CAD build for the part. Positions are in the model's coordinates, mm. Give positions to 0.01 mm unless a question says otherwise; leave off trailing zeros. Write each loop counter-clockwise with the first axis right and the second up, starting at its lowest first coordinate (ties: lowest second). Pieces come first, ordered by that corner, then holes. Notation, with made-up numbers: (43.25, 70) - (63.25, 70) arc R35 ccw to (63.25, 104) - close; hole circle Ø7 at (74.5, -21.75). An arc over 180 degrees is marked (long way). Answer as a JSON object with one key per item and string values.
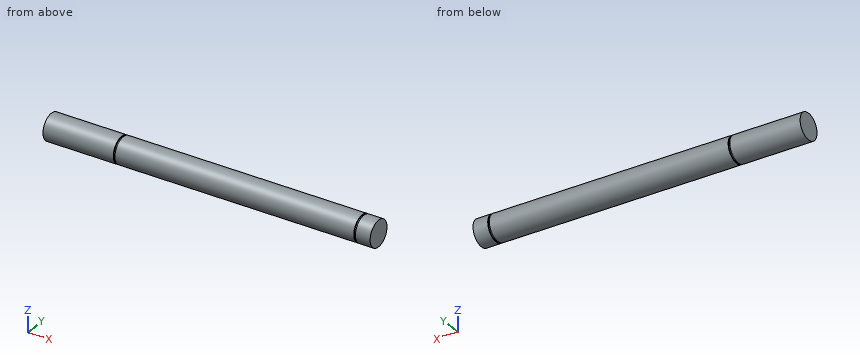
from build123d import *

# Parameters (mm, degrees)
SKETCH1_R           = 4
BOSS_EXTRUDE1_DEPTH = 50
SKETCH2_W           = 0.5
SKETCH2_H           = 0.3
SKETCH3_W           = 0.5
SKETCH3_H           = 0.3


with BuildPart() as part:
    # Sketch1 → Boss-Extrude1 (new, symmetric)
    with BuildSketch(Plane(origin=(0, 0, 0), x_dir=(0, 0, -1), z_dir=(1, 0, 0))):
        Circle(SKETCH1_R)
    extrude(amount=BOSS_EXTRUDE1_DEPTH, both=True)

    # Sketch2 → Cut-Revolve1 (revolve, cut)
    with BuildSketch(Plane.XY, mode=Mode.PRIVATE) as cut_revolve1_sk:
        with Locations((45.25, 3.85)):
            Rectangle(SKETCH2_W, SKETCH2_H)
    revolve(cut_revolve1_sk.sketch.rotate(Axis((0, 0, 0), (1, 0, 0)), 90), axis=Axis((0, 0, 0), (1, 0, 0)), mode=Mode.SUBTRACT)

    # Sketch3 → Cut-Revolve2 (revolve, cut)
    with BuildSketch(Plane.XY, mode=Mode.PRIVATE) as cut_revolve2_sk:
        with Locations((-28.25, 3.85)):
            Rectangle(SKETCH3_W, SKETCH3_H)
    revolve(cut_revolve2_sk.sketch.rotate(Axis((0, 0, 0), (-1, 0, 0)), 270), axis=Axis((0, 0, 0), (-1, 0, 0)), mode=Mode.SUBTRACT)


solid = part.part
(1) Flat gauge pin, fed straight in: P1, Ø1, axis at x = 28.5, z = -2, coming from the -Y side. Where does the tip first touch, or does it go through?
Answer key:
{"P1": "stops at y = -3.71"}
(2) Saw through at A-A, the plane y = -1.5. Give the cut face in (x, z), and give its area (3 significant figures).
Answer key:
{"outline": "(-50, -3.71) - (-28.5, -3.71) - (-28.5, -3.38) - (-28, -3.38) - (-28, -3.71) - (45, -3.71) - (45, -3.38) - (45.5, -3.38) - (45.5, -3.71) - (50, -3.71) - (50, 3.71) - (45.5, 3.71) - (45.5, 3.38) - (45, 3.38) - (45, 3.71) - (-28, 3.71) - (-28, 3.38) - (-28.5, 3.38) - (-28.5, 3.71) - (-50, 3.71) - close", "area": "741 mm²"}
(3) Probe L1, parallel to X at y = -1, z = 3.75; L2, parallel to Z at x = -38.5, y = 0.25; L3, parallel to Z at x = 38, y = -1.5. List the from-to ranges inside material, lowest first. Write a range as [from, to].
Answer key:
{"L1": "x = [-50, -28.5], [-28, 45], [45.5, 50]", "L2": "z = [-3.99, 3.99]", "L3": "z = [-3.71, 3.71]"}
(4) Saw through at B-B, the plane z = -1.75. Give the cut face in (x, y).
Answer key:
{"outline": "(-50, -3.6) - (-28.5, -3.6) - (-28.5, -3.26) - (-28, -3.26) - (-28, -3.6) - (45, -3.6) - (45, -3.26) - (45.5, -3.26) - (45.5, -3.6) - (50, -3.6) - (50, 3.6) - (45.5, 3.6) - (45.5, 3.26) - (45, 3.26) - (45, 3.6) - (-28, 3.6) - (-28, 3.26) - (-28.5, 3.26) - (-28.5, 3.6) - (-50, 3.6) - close"}
(5) Saw through at C-C, the plane x = 41. Give the cut face in (y, z), and give its area (3 significant figures).
Answer key:
{"outline": "circle Ø8 at (0, 0)", "area": "50.3 mm²"}
